from build123d import *

# Parameters (mm, degrees)
F0_W      = 100
F0_H      = 100
F1_DEPTH  = 2000
F2_W      = 200
F2_H      = 200
F3_DEPTH  = 12
F5_DEPTH  = 150
F7_DEPTH  = 20
F8_W      = 200
F8_H      = 200
F9_DEPTH  = 3
F11_DEPTH = 100
F13_R     = 25


with BuildPart() as f1:
    # F0 (on Top) → F1 (new body)
    with BuildSketch(Plane.XY):
        Rectangle(F0_W, F0_H)
    extrude(amount=F1_DEPTH)

    # F2 (on face) → F3 (join)
    with BuildSketch(Plane(origin=(0, 0, 0), x_dir=(1, 0, 0), z_dir=(0, 0, -1))):
        Rectangle(F2_W, F2_H)
    extrude(amount=F3_DEPTH)

    # F4 (on face) → F5 (join)
    with BuildSketch(Plane(origin=(0, 0, -12), x_dir=(1, 0, 0), z_dir=(0, 0, -1))):
        with BuildLine():
            ThreePointArc((-75, 85), (-82.0710678119, 67.9289321881), (-65, 75))
            ThreePointArc((-65, 75), (-67.9289321881, 82.0710678119), (-75, 85))
        make_face()
        with BuildLine():
            ThreePointArc((75, 85), (67.9289321881, 67.9289321881), (85, 75))
            ThreePointArc((85, 75), (82.0710678119, 82.0710678119), (75, 85))
        make_face()
        with BuildLine():
            ThreePointArc((-75, -85), (-67.9289321881, -82.0710678119), (-65, -75))
            ThreePointArc((-65, -75), (-82.0710678119, -67.9289321881), (-75, -85))
        make_face()
        with BuildLine():
            ThreePointArc((75, -85), (82.0710678119, -82.0710678119), (85, -75))
            ThreePointArc((85, -75), (67.9289321881, -67.9289321881), (75, -85))
        make_face()
    extrude(amount=F5_DEPTH)

    # F6 (on face) → F7 (join)
    with BuildSketch(Plane.XY):
        with BuildLine():
            ThreePointArc((-65, 75), (-67.9289321881, 82.0710678119), (-75, 85))
            Line((-75, 85), (-75, 75))
            Line((-75, 75), (-75, 65))
            ThreePointArc((-75, 65), (-67.9289321881, 67.9289321881), (-65, 75))
        make_face()
        with BuildLine():
            ThreePointArc((-65, -75), (-67.9289321881, -67.9289321881), (-75, -65))
            ThreePointArc((-75, -65), (-82.0710678119, -82.0710678119), (-65, -75))
        make_face()
        with BuildLine():
            Line((-75, 75), (-75, 85))
            ThreePointArc((-75, 85), (-85, 75), (-75, 65))
            Line((-75, 65), (-75, 75))
        make_face()
        with BuildLine():
            ThreePointArc((85, 75), (82.0710678119, 82.0710678119), (75, 85))
            Line((75, 85), (75, 75))
            Line((75, 75), (75, 65))
            ThreePointArc((75, 65), (82.0710678119, 67.9289321881), (85, 75))
        make_face()
        with BuildLine():
            ThreePointArc((85, -75), (82.0710678119, -67.9289321881), (75, -65))
            ThreePointArc((75, -65), (67.9289321881, -82.0710678119), (85, -75))
        make_face()
        with BuildLine():
            Line((75, 75), (75, 85))
            ThreePointArc((75, 85), (65, 75), (75, 65))
            Line((75, 65), (75, 75))
        make_face()
    extrude(amount=F7_DEPTH)

    # F8 (on face) → F9 (join)
    with BuildSketch(Plane(origin=(0, 0, -162), x_dir=(1, 0, 0), z_dir=(0, 0, -1))):
        Rectangle(F8_W, F8_H)
    extrude(amount=F9_DEPTH)

    # F10 (on face) → F11 (join)
    with BuildSketch(Plane(origin=(0, 0, -165), x_dir=(1, 0, 0), z_dir=(0, 0, -1))):
        with BuildLine():
            ThreePointArc((-65, 75), (-67.9289321881, 82.0710678119), (-75, 85))
            Line((-75, 85), (-75, 75))
            Line((-75, 75), (-75, 65))
            ThreePointArc((-75, 65), (-67.9289321881, 67.9289321881), (-65, 75))
        make_face()
        with BuildLine():
            ThreePointArc((85, 75), (67.9289321881, 82.0710678119), (75, 65))
            ThreePointArc((75, 65), (82.0710678119, 67.9289321881), (85, 75))
        make_face()
        with BuildLine():
            ThreePointArc((75, -65), (67.9289321881, -67.9289321881), (65, -75))
            Line((65, -75), (75, -75))
            Line((75, -75), (75, -65))
        make_face()
        with BuildLine():
            Line((75, -75), (65, -75))
            ThreePointArc((65, -75), (75, -85), (85, -75))
            ThreePointArc((85, -75), (82.0710678119, -67.9289321881), (75, -65))
            Line((75, -65), (75, -75))
        make_face()
        with BuildLine():
            ThreePointArc((-65, -75), (-67.9289321881, -67.9289321881), (-75, -65))
            Line((-75, -65), (-75, -75))
            Line((-75, -75), (-65, -75))
        make_face()
        with BuildLine():
            Line((-75, -75), (-75, -65))
            ThreePointArc((-75, -65), (-82.0710678119, -82.0710678119), (-65, -75))
            Line((-65, -75), (-75, -75))
        make_face()
        with BuildLine():
            Line((-75, 75), (-75, 85))
            ThreePointArc((-75, 85), (-85, 75), (-75, 65))
            Line((-75, 65), (-75, 75))
        make_face()
    extrude(amount=F11_DEPTH)

    # F14: sweep along a path in F12
    with BuildLine(Plane.XZ) as f14_path:
        Line((-823.6663937569, 0), (-50.3681525588, 431.6245317459))
    # F13 (on face) → F14 (sweep)
    with BuildSketch(Plane(origin=(-50, 0, 0), x_dir=(0, -1, 0), z_dir=(-1, 0, 0))):
        with Locations((0, 431.8528473377)):
            Circle(F13_R)
    sweep(path=f14_path.line)


solid = f1.part
Design review of the part built by this model. Coordinates are the model's own, in mm. A direction names the side the tool comes from. Round coordinates to 2 decimals unless told otherwise and drop trailing zeros. Order: outer loops, then holes, each group sorted by start corner. A loop starts at its lowest first (then second) coordinate and runs counter-clockwise, first axis right, second up.
1) Consider section C-C (z = 1830). State the section outline as (x, y) points, plus the area to 3 significant figures.
The answers:
outline: (-50, -50) - (50, -50) - (50, 50) - (-50, 50) - close
area: 10,000 mm2
2) Machinability: for faces 5 (the flat face through (-1, -1, -165)), 6 (the flat face through (-1, -1, -12)), 7 (the flat face through (-1, 50, 986)), which of the approach directions +Z, -Z, +X, -X, +Y, -Y give a long, thin tool a straight path to every point of the face, cutting with its end or side? Answer none if there is none.
The answers:
face 5: -Z
face 6: none
face 7: +Z, +X, -X, +Y
3) Consider section B-B (z = -57.5). State the section outline as (x, y) points, plus the area to 3 significant figures.
The answers:
outline: circle Ø20 at (-75, -75); circle Ø20 at (-75, 75); circle Ø20 at (75, -75); circle Ø20 at (75, 75)
area: 1,260 mm2
4) Draft analysis for pull direction X (two halves, no side actions). For faces 1 (the flat face through (50, -1, 986)), 2 (the flat face through (-823.298, 0, 1)), 3 (the flat face through (-50, -1, 986)), 4 (the flat face through (-1, -50, 986)), state which applies: released by +X, released by -X, zero draft, split by the parting line, or undercut.
The answers:
face 1: released by +X
face 2: released by -X
face 3: undercut
face 4: zero draft
5) Clearance check with flat-ended pins moving along their axes: pin 1 Ø8 at (y, z) = (-25.5, 1473.5) entering from +X; pin 2 Ø3 at (y, z) = (-34.5, 789.5) entering from -X; pin 3 Ø6 at (x, y) = (-80, -75) entering from +Z. State where each tip first meets the part, or that it passes through.
The answers:
pin 1: stops at x = 50
pin 2: stops at x = -50
pin 3: stops at z = 20
6) Consider section A-A (x = 23.5). State the section outline as (y, z) points, plus the area to 3 significant figures.
The answers:
outline: (-100, -165) - (100, -165) - (100, -162) - (-100, -162) - close; (-100, -12) - (100, -12) - (100, 0) - (50, 0) - (50, 2000) - (-50, 2000) - (-50, 0) - (-100, 0) - close
area: 203,000 mm2
7) For L1, parallel to Y at x = -35.5, z = 1050; L2, parallel to Z at x = -10.5, y = 43, list the stretches that pass through material, from the lowest coordinate up.
The answers:
L1: y = -50 to 50
L2: z = -165 to -162, -12 to 2000
